Can you work these out from the model? Positions are in its coordinate system, mm. A direction names the side the tool comes from. Give positions to 0.01 mm unless a question says otherwise; leave off trailing zeros. Order: outer loops, then holes, each group sorted by start corner. A loop starts at its lowest first (then second) coordinate and runs counter-clockwise, first axis right, second up. Notation, with made-up numbers: M 11.5,67.5 L 20.5,67.5 A21 cw 20.5,106.5 Z; hole C 36.25,76 d10. An arc over 180 degrees is marked long. Write each question's results on one line, items separated by ' | '.
from build123d import *

# Parameters (mm, degrees)
F1_DEPTH      = 11.43
F1_DEPTH_BACK = 11.43
F4_DEPTH      = 25.4
F5_DEPTH      = 25.4
F6_R          = 9.525
F7_R          = 3.175


with BuildPart() as f1:
    # F0 (on Front) → F1 (new body, two sides)
    with BuildSketch(Plane.XZ) as f1_sk:
        with BuildLine():
            Line((44.7153352637, 32.1372644044), (12.5878580118, -9.6727170782))
            ThreePointArc((12.5878580118, -9.6727170782), (9.1419703563, -12.9784437821), (4.868931841, -15.1099016452))
            Line((4.868931841, -15.1099016452), (6.2711842112, -19.461553319))
            Line((6.2711842112, -19.461553319), (69.7327711211, 0.987960413))
            Line((69.7327711211, 0.987960413), (67.7851983847, 7.0319210711))
            Line((67.7851983847, 7.0319210711), (46.8382920625, 0.2821048541))
            Line((46.8382920625, 0.2821048541), (40.7535190047, 19.1651628715))
            Line((40.7535190047, 19.1651628715), (48.4916926673, 29.235449281))
            Line((48.4916926673, 29.235449281), (44.7153352637, 32.1372644044))
        make_face()
    extrude(amount=F1_DEPTH)
    extrude(f1_sk.sketch, amount=-F1_DEPTH_BACK)

    # F3 (on face) → F4 (cut)
    with BuildSketch(Plane(origin=(16.3642154154, 0, -12.5745322016), x_dir=(0, 1, 0), z_dir=(0.7929359378, 0, -0.6093050128))):
        with BuildLine():
            ThreePointArc((-2.54, 49.5530698125), (0, 47.0130698125), (2.54, 49.5530698125))
            ThreePointArc((2.54, 49.5530698125), (0, 52.0930698125), (-2.54, 49.5530698125))
        make_face()
        with BuildLine():
            ThreePointArc((-2.54, 49.5530698125), (0, 52.0930698125), (2.54, 49.5530698125))
            Line((2.54, 49.5530698125), (2.54, 52.7280698125))
            Line((2.54, 52.7280698125), (-2.54, 52.7280698125))
            Line((-2.54, 52.7280698125), (-2.54, 49.5530698125))
        make_face()
    extrude(amount=-F4_DEPTH, mode=Mode.SUBTRACT)

    # F2 (on face) → F5 (cut)
    with BuildSketch(Plane(origin=(4.3236114748, 0, -13.4175926609), x_dir=(0.951804828, 0, 0.3067043679), z_dir=(-0.3067043679, 0, 0.951804828))):
        with BuildLine():
            ThreePointArc((63.5, -2.54), (65.2960512242, -1.7960512242), (66.04, 0))
            ThreePointArc((66.04, 0), (65.2960512242, 1.7960512242), (63.5, 2.54))
            ThreePointArc((63.5, 2.54), (60.96, 0), (63.5, -2.54))
        make_face()
        with BuildLine():
            ThreePointArc((63.5, 2.54), (65.2960512242, 1.7960512242), (66.04, 0))
            ThreePointArc((66.04, 0), (65.2960512242, -1.7960512242), (63.5, -2.54))
            Line((63.5, -2.54), (66.675, -2.54))
            Line((66.675, -2.54), (66.675, 2.54))
            Line((66.675, 2.54), (63.5, 2.54))
        make_face()
    extrude(amount=-F5_DEPTH, mode=Mode.SUBTRACT)

    # F6
    f6_edges = [f1.edges().sort_by_distance(p)[0] for p in [
        (46.838292, 0, 0.282105),
        (40.753519, 0, 19.165163),
    ]]
    fillet(f6_edges, radius=F6_R)

    # F7
    f7_edges = [f1.edges().sort_by_distance(p)[0] for p in [
        (4.868932, 0, -15.109902),
    ]]
    fillet(f7_edges, radius=F7_R)


solid = f1.part
(1) Imagine slicing it at C-C, the plane x = 18. Write out the boundary of the cut face in (y, z), plus the area to 3 significant figures.
Data:
outline: M -11.43,-15.68 L 11.43,-15.68 L 11.43,-2.63 L -11.43,-2.63 Z | area: 298 mm2
(2) For faces 1 (the face through (48.731, -0.16, 3.746)), 2 (the face through (46, -2.54, 29)), 3 (the face through (43.114, -0.16, 11.841)), 4 (the face through (35, -11.43, 1)), 5 (the face through (68.77, -7.05, 3.97)), which set-ups out of +Z, -Z, +X, -X, +Y, -Y let a thin tool reach every point of the face, with its end or its side?
Data:
face 1: +Y, -Y | face 2: +Z, +X | face 3: +X, +Y, -Y | face 4: +Z, -Z, +X, -X, -Y | face 5: +Z, +X, +Y, -Y
(3) Will these pins go through, and if not, where does the flat tip stop? P1, Ø5, axis at x = 61, y = 6, coming from the -Z side; P2, Ø1, axis at x = 19, y = 2.5, coming from the +Z side; P3, Ø6, axis at x = 31.5, y = -8, coming from the -Z side.
Data:
P1: stops at z = -2.63 | P2: stops at z = -0.68 | P3: stops at z = -12.3
(4) We'd pull the mould along X, two halves only. Please class faces 6 (the face through (28.876, -0.16, 11.525)), 7 (the face through (37.56, -0.16, -9.38)), 8 (the face through (61.928, -0.16, 5.144)): +X half, -X half, draft (parallel to the pull), parting line (faces both ways), or undercut.
Data:
face 6: -X half | face 7: +X half | face 8: undercut
(5) Imagine slicing it at B-B, the plane z = -12.5. Write out the boundary of the cut face in (x, y).
Data:
outline: M 9.79,-11.43 L 27.88,-11.43 L 27.88,11.43 L 9.79,11.43 Z
(6) I need wall thicknesses on L1, parallel to X at y = 7.75, z = 11; L2, parallel to X at y = 10, z = 18; L3, parallel to Z at x = 15.5, y = 7.25. Which ranges of each line are inside material? Lowest first, please. Write a range as from..to.
Data:
L1: x = 28.47..43.38 | L2: x = 33.85..41.85 | L3: z = -16.49..-5.88
